```python
from build123d import *

# Parameters (mm, degrees)
BOSS_EXTRUDE1_DEPTH = 20
BOSS_EXTRUDE2_DEPTH = 20
FILLET1_R           = 19
FILLET2_R           = 10
SKETCH3_R           = 5
SKETCH3_R_2         = 10
CUT_EXTRUDE1_DEPTH  = 590.788097561
SKETCH4_W           = 120
SKETCH4_H           = 120
BOSS_EXTRUDE3_DEPTH = 10
FILLET3_R           = 10
CUT_EXTRUDE2_DEPTH  = 10


with BuildPart() as part:
    # Sketch1 → Boss-Extrude1 (new body)
    with BuildSketch(Plane.XY):
        with BuildLine():
            Line((-75, 500), (-75, 173.205080757))
            ThreePointArc((-75, 173.205080757), (-82.846215434, 117.735061134), (-105.769230769, 66.617338753))
            ThreePointArc((-105.769230769, 66.617338753), (0, -125), (105.769230769, 66.617338753))
            ThreePointArc((105.769230769, 66.617338753), (82.846215434, 117.735061134), (75, 173.205080757))
            Line((75, 173.205080757), (75, 500))
            ThreePointArc((75, 500), (0, 575), (-75, 500))
        make_face()
    extrude(amount=BOSS_EXTRUDE1_DEPTH)

    # Sketch2 → Boss-Extrude2 (add)
    with BuildSketch(Plane(origin=(0, 0, 0), x_dir=(-1, 0, 0), z_dir=(0, 0, -1))):
        with BuildLine():
            Line((-55, 500), (-55, 173.205080757))
            ThreePointArc((-55, 173.205080757), (-63.630836977, 112.188059172), (-88.846153846, 55.958564552))
            ThreePointArc((-88.846153846, 55.958564552), (0, -105), (88.846153846, 55.958564552))
            ThreePointArc((88.846153846, 55.958564552), (63.630836977, 112.188059172), (55, 173.205080757))
            Line((55, 173.205080757), (55, 500))
            ThreePointArc((55, 500), (0, 555), (-55, 500))
        make_face()
    extrude(amount=BOSS_EXTRUDE2_DEPTH)

    # Fillet1
    fillet1_edges = [part.edges().sort_by_distance(p)[0] for p in [
        (0, 555, 0),
        (55, 336.602540378, 0),
        (63.630836977, 112.188059172, 0),
        (0, -105, 0),
        (-63.630836977, 112.188059172, 0),
        (-55, 336.602540378, 0),
    ]]
    fillet(fillet1_edges, radius=FILLET1_R)

    # Fillet2
    fillet2_edges = [part.edges().sort_by_distance(p)[0] for p in [
        (-82.846215434, 117.735061134, 20),
        (0, -125, 20),
        (82.846215434, 117.735061134, 20),
        (75, 336.602540378, 20),
        (0, 575, 20),
        (-75, 336.602540378, 20),
    ]]
    fillet(fillet2_edges, radius=FILLET2_R)

    # Sketch3 → Cut-Extrude1 (cut, through all)
    with BuildSketch(Plane.XY.offset(20)):
        with Locations((-32.5, 500)):
            Circle(SKETCH3_R)
        with Locations((-16.25, 528.145825623)):
            Circle(SKETCH3_R)
        with Locations((16.25, 528.145825623)):
            Circle(SKETCH3_R)
        with Locations((32.5, 500)):
            Circle(SKETCH3_R)
        with Locations((16.25, 471.854174377)):
            Circle(SKETCH3_R)
        with Locations((-16.25, 471.854174377)):
            Circle(SKETCH3_R)
        with Locations((-45, 0)):
            Circle(SKETCH3_R_2)
        with Locations((0, 45)):
            Circle(SKETCH3_R_2)
        with Locations((45, 0)):
            Circle(SKETCH3_R_2)
        with Locations((0, -45)):
            Circle(SKETCH3_R_2)
    extrude(amount=-CUT_EXTRUDE1_DEPTH, mode=Mode.SUBTRACT)

    # Sketch4 → Boss-Extrude3 (add)
    with BuildSketch(Plane.XY.offset(20)):
        with Locations((0, 325)):
            Rectangle(SKETCH4_W, SKETCH4_H)
    extrude(amount=BOSS_EXTRUDE3_DEPTH)

    # Fillet3
    fillet3_edges = [part.edges().sort_by_distance(p)[0] for p in [
        (60, 265, 25),
        (60, 385, 25),
        (-60, 385, 25),
        (-60, 265, 25),
    ]]
    fillet(fillet3_edges, radius=FILLET3_R)

    # Sketch5 → Cut-Extrude2 (cut)
    with BuildSketch(Plane.XY.offset(30)):
        with BuildLine():
            Line((31, 275), (-31, 275))
            ThreePointArc((-31, 275), (-44.435028843, 280.564971157), (-50, 294))
            Line((-50, 294), (-50, 356))
            ThreePointArc((-50, 356), (-44.435028843, 369.435028843), (-31, 375))
            Line((-31, 375), (31, 375))
            ThreePointArc((31, 375), (44.435028843, 369.435028843), (50, 356))
            Line((50, 356), (50, 294))
            ThreePointArc((50, 294), (44.435028843, 280.564971157), (31, 275))
        make_face()
    extrude(amount=-CUT_EXTRUDE2_DEPTH, mode=Mode.SUBTRACT)


solid = part.part
```
The model under review builds one solid part; all positions refer to its coordinate system, in mm. A direction names the side the tool comes from. Give positions to 0.01 mm unless a question says otherwise; leave off trailing zeros. Loops run counter-clockwise (first coordinate to the right, second up) from the corner with the lowest first, then second, coordinate; pieces in that order, holes last. Notation, with made-up numbers: (10, -10) -> (63, -10) arc R9 cw to (63, -2) -> close; hole circle Ø11 at (33.25, 15). An arc over 180 degrees is marked (long way). Use CSV: the item, a comma, the result in double quotes.
1. For P1, Ø11, axis at y = 313.5, z = 23, coming from the -X side; P2, Ø4, axis at x = -54, z = 7, coming from the +Y side; P3, Ø5, axis at y = 326, z = 3, coming from the -X side, all flat-tipped, find the tip position at first contact; note any pin that passes through.
Result:
P1,"stops at x = -71.61"
P2,"stops at y = 554.05"
P3,"stops at x = -75"
2. Machinability: for faces 1 (the face through (44.58, 280.71, 25.07)), 2 (the face through (-60.71, 338.89, -5.42)), 3 (the face through (-1.209, 554.987, -19.493)), which of the approach directions +Z, -Z, +X, -X, +Y, -Y give a long, thin tool a straight path to every point of the face, cutting with its end or side? Answer none if there is none.
Result:
face 1,"+Z"
face 2,"-Z, -X, +Y"
face 3,"-Z, +Y"
3. Consider section A-A, the plane y = 485. Write out the cut boundary in (x, z).
Result:
outline,"(-75, 0) -> (-74, 0) arc R19 cw to (-55, -19) -> (-55, -20) -> (55, -20) -> (55, -19) arc R19 cw to (74, 0) -> (75, 0) -> (75, 10) arc R10 ccw to (65, 20) -> (-65, 20) arc R10 ccw to (-75, 10) -> close"
4. To check wall thickness, follow probe 1 along Y at (x, z) = (0, 8); probe 2 along Y at (x, z) = (16, 7); probe 3 along X at (y, z) = (7, -4). State the ranges of each line that lie inside material, in increasing order. Write a range as from..to.
Result:
probe 1,"y = -125..-55, -35..35, 55..575"
probe 2,"y = -123.97..466.86, 476.85..523.15, 533.14..573.27"
probe 3,"x = -112.12..-52.14, -37.86..37.86, 52.14..112.12"
5. Consider section B-B, the plane z = -13. Count the separate pieces of the cut face and the enclosed holes in it, then the cut area to 3 significant figures.
Result:
separate pieces,"1"
enclosed holes,"10"
area,"84,400 mm²"
6. The part is to be moulded in two halves that separate along X. For faces 4 (the face through (-3.732, -124.944, 4.93)), 5 (the face through (-63.87, 111.36, -19.49)), 6 (the face through (-2.17, -54.76, 0.28)), say which applies: +X half, -X half, draft (parallel to the pull), parting line (faces both ways), or undercut.
Result:
face 4,"parting line"
face 5,"-X half"
face 6,"undercut"
